Autodesk Inventor part; units mm, degrees
ref_plane "YZ Plane" through (0, 0, 0) normal (1, 0, 0) x (0, 1, 0)
ref_plane "XZ Plane" through (0, 0, 0) normal (0, 1, 0) x (-1, 0, 0)
ref_plane "XY Plane" through (0, 0, 0) normal (0, 0, 1) x (1, 0, 0)
sketch "Sketch1" plane through (0, 0, 0) normal (0, 0, 1) x (1, 0, 0)
  line L0 (-5.0917, 19.05) -> (-5.0917, 25.4)
  line L1 (0, 25.4) -> (-5.0917, 25.4)
  line L2 (-18.4964, 0) -> (0, 0)
  line L3 (0, 25.4) -> (0, 0)
  arc A0 (-12.7, 6.35) -> (-5.0917, 19.05) centre (-19.7746, 19.2173) ccw
  spline S0 degree 2 poles (-12.7, 6.35) (-18.092, 3.6812) (-18.4964, 0) knots 0 0 0 1 1 1
  point P0 (-17.2168, 2.9909)
  dimension "d1" = 6.35
  dimension "d7" = 25.4
  dimension "d8" = 18.4964
extrude "Extrusion1" add sketch "Sketch1" along normal blind 177.8
hole "Hole1" at (0, 21.4671, 171.3774) direction (-1, 0, 0) diameter 4 end through all
pattern_linear "Rectangular Pattern1" count 4 spacing 53.848 along (0, 0, -1) of "Hole1"
properties part number "Intake inclined edge bottom"
Geometry check sheet. Reference: the model listing, model coordinates, mm. A direction names the side the tool comes from. Give positions to 0.01 mm unless a question says otherwise; leave off trailing zeros. Write each loop counter-clockwise with the first axis right and the second up, starting at its lowest first coordinate (ties: lowest second). Pieces come first, ordered by that corner, then holes. Notation, with made-up numbers: (68.5, 36.5) - (92.5, 36.5) arc R10 cw to (92.5, 51.5) - close; hole circle Ø6 at (75, 69.5). An arc over 180 degrees is marked (long way). Put each result on its own line as item: value.
1. Sectioned sample at B-B, the plane x = -11. Enter the section's corners in (y, z), plus the area to 3 significant figures.
Ans:
outline: (0, 0) - (7.44, 0) - (7.44, 177.8) - (0, 177.8) - close
area: 1,320 mm²
2. Sectioned sample at A-A, the plane y = 8. Enter the section's corners in (x, z).
Ans:
outline: (-10.3, 0) - (0, 0) - (0, 177.8) - (-10.3, 177.8) - close
3. Go/stop test with flat-tipped pins: pin 1 (8 mm diameter, centred on y = 17.5, z = 26, fed in from +X); pin 2 (1.9 mm diameter, centred on y = 22.5, z = 80, fed in from -X); pin 3 (1 mm diameter, centred on y = 17, z = 34, fed in from -X); pin 4 (4 mm diameter, centred on x = -14, z = 74, fed in from +Y). Record where each tip stops, or that it passes through.
Ans:
pin 1: stops at x = 0
pin 2: stops at x = -5.09
pin 3: stops at x = -5.34
pin 4: stops at y = 6.76
4. Set-up check for faces 1 (the flat face through (-3, 25.4, 88)), 2 (the flat face through (-5.092, 22, 88)): record each of +Z, -Z, +X, -X, +Y, -Y from which the full face is reachable in a straight line by a thin tool's end or side.
Ans:
face 1: +Z, -Z, +X, -X, +Y
face 2: +Z, -Z, -X, +Y
5. Thickness scan on line 1 (X direction, y = 23.75, z = 156.5); line 2 (X direction, y = 1.75, z = 124.5); line 3 (Y direction, x = -8.75, z = 107.5). Record the ranges inside material, lowest first.
Ans:
line 1: x = -5.09 to 0
line 2: x = -18 to 0
line 3: y = 0 to 9.52
6. Draft check along Z on faces 3 (the flat face through (-5, 10, 177.8)), 4 (the flat face through (0, 13, 88)), 5 (the cylindrical face through (-2.58, 22.68, 119.12)), 6 (the cylindrical face through (-2.58, 21.38, 65.68)). Enter one of: +Z half, -Z half, draft (parallel to the pull), parting line (faces both ways), or undercut.
Ans:
face 3: +Z half
face 4: draft
face 5: undercut
face 6: undercut
